from build123d import *

# Parameters (mm, degrees)
SKETCH1_R           = 40
SKETCH1_R_2         = 8
BOSS_EXTRUDE1_DEPTH = 4
SKETCH2_R           = 2.5
CUT_EXTRUDE1_DEPTH  = 4
SKETCH3_R           = 2
CUT_EXTRUDE2_DEPTH  = 4


with BuildPart() as part:
    # Sketch1 → Boss-Extrude1 (new body)
    with BuildSketch(Plane.XY):
        Circle(SKETCH1_R)
        Circle(SKETCH1_R_2, mode=Mode.SUBTRACT)
    extrude(amount=BOSS_EXTRUDE1_DEPTH)

    # Sketch2 → Cut-Extrude1 (cut)
    with BuildSketch(Plane.XY.offset(4)):
        with Locations((0, 35)):
            Circle(SKETCH2_R)
        with Locations((18.922428611, 29.443873649)):
            Circle(SKETCH2_R)
        with Locations((31.837119837, 14.539525455)):
            Circle(SKETCH2_R)
        with Locations((34.643750466, -4.98101934)):
            Circle(SKETCH2_R)
        with Locations((26.451235102, -22.920125688)):
            Circle(SKETCH2_R)
        with Locations((9.860639489, -33.582254077)):
            Circle(SKETCH2_R)
        with Locations((-9.860639489, -33.582254077)):
            Circle(SKETCH2_R)
        with Locations((-26.451235102, -22.920125688)):
            Circle(SKETCH2_R)
        with Locations((-34.643750466, -4.98101934)):
            Circle(SKETCH2_R)
        with Locations((-31.837119837, 14.539525455)):
            Circle(SKETCH2_R)
        with Locations((-18.922428611, 29.443873649)):
            Circle(SKETCH2_R)
    extrude(amount=-CUT_EXTRUDE1_DEPTH, mode=Mode.SUBTRACT)

    # Sketch3 → Cut-Extrude2 (cut)
    with BuildSketch(Plane.XY.offset(4)):
        with Locations((0, 15)):
            Circle(SKETCH3_R)
        with Locations((15, 0)):
            Circle(SKETCH3_R)
        with Locations((0, -15)):
            Circle(SKETCH3_R)
        with Locations((-15, 0)):
            Circle(SKETCH3_R)
    extrude(amount=-CUT_EXTRUDE2_DEPTH, mode=Mode.SUBTRACT)


solid = part.part
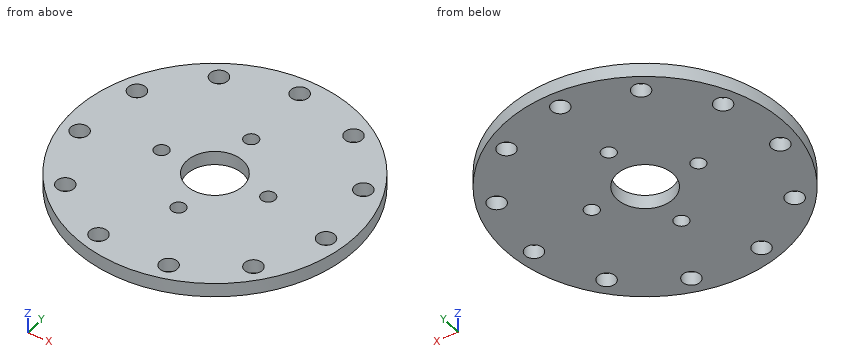
The listing builds one solid part. Answer for the finished solid, in the listing's coordinates (mm). Give positions to 0.01 mm unless a question says otherwise; leave off trailing zeros. Write each loop counter-clockwise with the first axis right and the second up, starting at its lowest first coordinate (ties: lowest second). Pieces come first, ordered by that corner, then holes.
Item 1: Section D-D, the plane x = 15 is taken. Write down the section's boundary in (y, z).
Item 2: Section C-C, the plane y = 7 is taken. Write down the section's boundary in (x, z).
Item 3: Section B-B, the plane y = -6.5 is taken. Write down the section's boundary in (x, z), plus the area to 3 significant figures.
Item 4: Find the intervals of material crossed by line 1 along X through (y, z) = (31.5, 2.75); line 2 along X through (y, z) = (-1.5, 3.1); line 3 along X through (y, z) = (14, 3.2), in increasing order.
Item 5: Section A-A, the plane x = 0 is taken. Write down the section's boundary in (y, z), plus the area to 3 significant figures.
Item 6: Flat-ended cylindrical pins translate along their axes: P1, Ø14.5, axis at x = 0, y = 0, coming from the +Z side; P2, Ø5, axis at x = -15, y = 0, coming from the -Z side; P3, Ø1.5, axis at y = -4.5, z = 2, coming from the +X side; P4, Ø1.5, axis at y = -27.5, z = 3.5, coming from the -X side. Find the tip coordinate at first contact, or state that the pin passes through.
Completed:
1. outline: (-37.08, 0) - (-2, 0) - (-2, 4) - (-37.08, 4) - close; (2, 0) - (37.08, 0) - (37.08, 4) - (2, 4) - close
2. outline: (-39.38, 0) - (-3.87, 0) - (-3.87, 4) - (-39.38, 4) - close; (3.87, 0) - (39.38, 0) - (39.38, 4) - (3.87, 4) - close
3. outline: (-39.47, 0) - (-36.63, 0) - (-36.63, 4) - (-39.47, 4) - close; (-32.66, 0) - (-4.66, 0) - (-4.66, 4) - (-32.66, 4) - close; (4.66, 0) - (32.66, 0) - (32.66, 4) - (4.66, 4) - close; (36.63, 0) - (39.47, 0) - (39.47, 4) - (36.63, 4) - close
3. area: 247 mm2
4. line 1: x = -24.65 to -20.34, -17.5 to 17.5, 20.34 to 24.65
4. line 2: x = -39.97 to -16.32, -13.68 to -7.86, 7.86 to 13.68, 16.32 to 39.97
4. line 3: x = -37.47 to -34.28, -29.4 to -1.73, 1.73 to 29.4, 34.28 to 37.47
5. outline: (-40, 0) - (-17, 0) - (-17, 4) - (-40, 4) - close; (-13, 0) - (-8, 0) - (-8, 4) - (-13, 4) - close; (8, 0) - (13, 0) - (13, 4) - (8, 4) - close; (17, 0) - (32.5, 0) - (32.5, 4) - (17, 4) - close; (37.5, 0) - (40, 0) - (40, 4) - (37.5, 4) - close
5. area: 204 mm2
6. P1: passes through
6. P2: stops at z = 0
6. P3: stops at x = 39.82
6. P4: stops at x = -29.74
